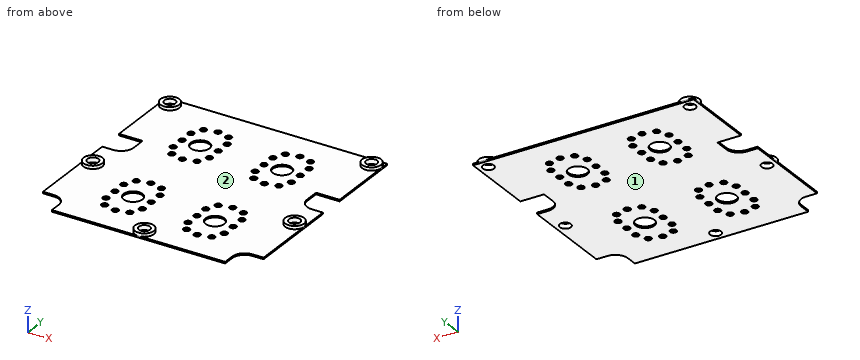
```python
from build123d import *

# Parameters (mm, degrees)
SKETCH1_W               = 70
SKETCH1_H               = 70
BOSS_EXTRUDE1_DEPTH     = 0.5
SKETCH2_R               = 3
CUT_EXTRUDE1_DEPTH      = 50.5
SKETCH3_R               = 1
CUT_EXTRUDE2_DEPTH      = 50.5
MIRROR2_COPY_1_SKETCH_R = 3
MIRROR2_COPY_1_DEPTH    = 50.5
MIRROR2_COPY_2_SKETCH_R = 1
MIRROR2_COPY_2_DEPTH    = 50.5
SKETCH4_R               = 3
BOSS_EXTRUDE2_DEPTH     = 1
SKETCH5_R               = 1.75
CUT_EXTRUDE3_DEPTH      = 50.520197899
SKETCH6_W               = 8.5
SKETCH6_H               = 8.5
CUT_EXTRUDE4_DEPTH      = 50.507575178
FILLET1_R               = 4
SKETCH7_R               = 3
BOSS_EXTRUDE3_DEPTH     = 1
SKETCH8_R               = 1.75
CUT_EXTRUDE5_DEPTH      = 50.520197899
FILLET1_OF_MIRROR3_R    = 4


with BuildPart() as part:
    # Sketch1 → Boss-Extrude1 (new body)
    with BuildSketch(Plane.XY):
        Rectangle(SKETCH1_W, SKETCH1_H)
    extrude(amount=BOSS_EXTRUDE1_DEPTH)

    # Sketch2 → Cut-Extrude1 (cut, through all)
    with BuildSketch(Plane.XY.offset(0.5)):
        with Locations((-13, 17)):
            Circle(SKETCH2_R)
    cut_extrude1 = extrude(amount=-CUT_EXTRUDE1_DEPTH, mode=Mode.SUBTRACT)

    # Sketch3 → Cut-Extrude2 (cut, through all)
    with BuildSketch(Plane.XY.offset(0.5)):
        with Locations((-7.25, 21.5)):
            Circle(SKETCH3_R)
        with Locations((-7.25, 17)):
            Circle(SKETCH3_R)
        with Locations((-7.25, 12.5)):
            Circle(SKETCH3_R)
        with Locations((-9, 9)):
            Circle(SKETCH3_R)
        with Locations((-9, 25)):
            Circle(SKETCH3_R)
        with Locations((-13, 26)):
            Circle(SKETCH3_R)
        with Locations((-13, 8)):
            Circle(SKETCH3_R)
        with Locations(Location((-17, 9, 0), (0, 0, 180))):
            Circle(SKETCH3_R)
        with Locations(Location((-18.75, 12.5, 0), (0, 0, 180))):
            Circle(SKETCH3_R)
        with Locations(Location((-18.75, 17, 0), (0, 0, 180))):
            Circle(SKETCH3_R)
        with Locations(Location((-18.75, 21.5, 0), (0, 0, 180))):
            Circle(SKETCH3_R)
        with Locations(Location((-17, 25, 0), (0, 0, 180))):
            Circle(SKETCH3_R)
    cut_extrude2 = extrude(amount=-CUT_EXTRUDE2_DEPTH, mode=Mode.SUBTRACT)

    # Mirror1: Cut-Extrude1, Cut-Extrude2 across plane
    add(cut_extrude1.mirror(Plane(origin=(0, 0, 0), x_dir=(0, 0, 1), z_dir=(1, 0, 0))), mode=Mode.SUBTRACT)
    add(cut_extrude2.mirror(Plane(origin=(0, 0, 0), x_dir=(0, 0, 1), z_dir=(1, 0, 0))), mode=Mode.SUBTRACT)

    # Mirror2: Cut-Extrude1, Cut-Extrude2 across plane
    add(cut_extrude1.mirror(Plane.ZX), mode=Mode.SUBTRACT)
    add(cut_extrude2.mirror(Plane.ZX), mode=Mode.SUBTRACT)

    # Mirror2 copy 1 sketch → Mirror2 copy 1 (cut, through all)
    with BuildSketch(Plane(origin=(0, 0, 0.5), x_dir=(-1, 0, 0), z_dir=(0, 0, 1))):
        with Locations((-13, 17)):
            Circle(MIRROR2_COPY_1_SKETCH_R)
    extrude(amount=-MIRROR2_COPY_1_DEPTH, mode=Mode.SUBTRACT)

    # Mirror2 copy 2 sketch → Mirror2 copy 2 (cut, through all)
    with BuildSketch(Plane(origin=(0, 0, 0.5), x_dir=(-1, 0, 0), z_dir=(0, 0, 1))):
        with Locations((-7.25, 21.5)):
            Circle(MIRROR2_COPY_2_SKETCH_R)
        with Locations((-7.25, 17)):
            Circle(MIRROR2_COPY_2_SKETCH_R)
        with Locations((-7.25, 12.5)):
            Circle(MIRROR2_COPY_2_SKETCH_R)
        with Locations((-9, 9)):
            Circle(MIRROR2_COPY_2_SKETCH_R)
        with Locations((-9, 25)):
            Circle(MIRROR2_COPY_2_SKETCH_R)
        with Locations((-13, 26)):
            Circle(MIRROR2_COPY_2_SKETCH_R)
        with Locations((-13, 8)):
            Circle(MIRROR2_COPY_2_SKETCH_R)
        with Locations(Location((-17, 9, 0), (0, 0, 180))):
            Circle(MIRROR2_COPY_2_SKETCH_R)
        with Locations(Location((-18.75, 12.5, 0), (0, 0, 180))):
            Circle(MIRROR2_COPY_2_SKETCH_R)
        with Locations(Location((-18.75, 17, 0), (0, 0, 180))):
            Circle(MIRROR2_COPY_2_SKETCH_R)
        with Locations(Location((-18.75, 21.5, 0), (0, 0, 180))):
            Circle(MIRROR2_COPY_2_SKETCH_R)
        with Locations(Location((-17, 25, 0), (0, 0, 180))):
            Circle(MIRROR2_COPY_2_SKETCH_R)
    extrude(amount=-MIRROR2_COPY_2_DEPTH, mode=Mode.SUBTRACT)

    # Sketch4 → Boss-Extrude2 (add)
    with BuildSketch(Plane.XY.offset(0.5)):
        with Locations(Location((-32, 32, 0), (0, 0, 180))):
            Circle(SKETCH4_R)
        with Locations(Location((-32, -7, 0), (0, 0, 180))):
            Circle(SKETCH4_R)
    boss_extrude2 = extrude(amount=BOSS_EXTRUDE2_DEPTH)

    # Sketch5 → Cut-Extrude3 (cut, through all)
    with BuildSketch(Plane.XY.offset(1.5)):
        with Locations((-32, 32)):
            Circle(SKETCH5_R)
        with Locations((-32, -7)):
            Circle(SKETCH5_R)
    cut_extrude3 = extrude(amount=-CUT_EXTRUDE3_DEPTH, mode=Mode.SUBTRACT)

    # Sketch6 → Cut-Extrude4 (cut, through all)
    with BuildSketch(Plane.XY.offset(0.5)):
        with Locations((-31.75, -31.75)):
            Rectangle(SKETCH6_W, SKETCH6_H)
        with Locations((-31.75, 6.75)):
            Rectangle(SKETCH6_W, SKETCH6_H)
    cut_extrude4 = extrude(amount=-CUT_EXTRUDE4_DEPTH, mode=Mode.SUBTRACT)

    # Fillet1
    fillet1_edges = [part.edges().sort_by_distance(p)[0] for p in [
        (-27.5, -27.5, 0.25),
        (-27.5, 2.5, 0.25),
    ]]
    fillet(fillet1_edges, radius=FILLET1_R)

    # Sketch7 → Boss-Extrude3 (add)
    with BuildSketch(Plane.XY.offset(0.5)):
        with Locations(Location((0, -32, 0), (0, 0, 270))):
            Circle(SKETCH7_R)
    extrude(amount=BOSS_EXTRUDE3_DEPTH)

    # Sketch8 → Cut-Extrude5 (cut, through all)
    with BuildSketch(Plane.XY.offset(1.5)):
        with Locations((0, -32)):
            Circle(SKETCH8_R)
    extrude(amount=-CUT_EXTRUDE5_DEPTH, mode=Mode.SUBTRACT)

    # Mirror3: Boss-Extrude2, Cut-Extrude3, Cut-Extrude4 across plane
    add(boss_extrude2.mirror(Plane(origin=(0, 0, 0), x_dir=(0, 0, 1), z_dir=(1, 0, 0))))
    add(cut_extrude3.mirror(Plane(origin=(0, 0, 0), x_dir=(0, 0, 1), z_dir=(1, 0, 0))), mode=Mode.SUBTRACT)
    add(cut_extrude4.mirror(Plane(origin=(0, 0, 0), x_dir=(0, 0, 1), z_dir=(1, 0, 0))), mode=Mode.SUBTRACT)

    # Fillet1 of Mirror3
    fillet1_of_mirror3_edges = [part.edges().sort_by_distance(p)[0] for p in [
        (27.5, -27.5, 0.25),
        (27.5, 2.5, 0.25),
    ]]
    fillet(fillet1_of_mirror3_edges, radius=FILLET1_OF_MIRROR3_R)


solid = part.part
```
Here's how the part is built. I have some questions about the finished solid (model axes, mm). Face numbers are marked on the shaded views. Give positions to 0.01 mm unless a question says otherwise; leave off trailing zeros. Write each loop counter-clockwise with the first axis right and the second up, starting at its lowest first coordinate (ties: lowest second). Pieces come first, ordered by that corner, then holes. Notation, with made-up numbers: (35, -2.5) -> (79, -2.5) arc R5 ccw to (79, 3.5) -> close; hole circle Ø5 at (-34.5, -18.5). An arc over 180 degrees is marked (long way). Use one line per item in the form item = value.
1) I'm going to push a flat-ended pin straight in: pin 1 (2.5 mm diameter, centred on x = 18.75, y = 17, fed in from +Z). Where does the tip first touch, or does it pass through?
Verdict:
pin_1 = 0.5
2) Suppose I cut it at A-A (x = -13). Please give me the cut outline in (y, z), and give its area (3 significant figures).
Verdict:
outline = (-35, 0) -> (-27, 0) -> (-27, 0.5) -> (-35, 0.5) -> close; (-25, 0) -> (-20, 0) -> (-20, 0.5) -> (-25, 0.5) -> close; (-14, 0) -> (-9, 0) -> (-9, 0.5) -> (-14, 0.5) -> close; (-7, 0) -> (7, 0) -> (7, 0.5) -> (-7, 0.5) -> close; (9, 0) -> (14, 0) -> (14, 0.5) -> (9, 0.5) -> close; (20, 0) -> (25, 0) -> (25, 0.5) -> (20, 0.5) -> close; (27, 0) -> (35, 0) -> (35, 0.5) -> (27, 0.5) -> close
area = 25.0 mm2
3) Suppose I cut it at C-C (z = 0.25). Give the number of separate pieces and of enclosed holes in the cut face, and give its area (3 significant figures).
Verdict:
separate_pieces = 1
enclosed_holes = 57
area = 4,360 mm2
4) If I drill on L1, parallel to Y at x = -32, z = 0.3; L2, parallel to Z at x = -16.5, y = -14; L3, parallel to X at y = -8, z = 1, over which ranges is the centre line in solid material (lowest first)? Write a range as [from, to].
Verdict:
L1 = [-27.5, -8.75], [-5.25, 2.5], [11, 30.25], [33.75, 35]
L2 = [0, 0.5]
L3 = [-34.83, -33.44], [-30.56, -29.17], [29.17, 30.56], [33.44, 34.83]
5) We'd pull the mould along X, two halves only. Please class the marked faces 1 and 2: +X half, -X half, draft (parallel to the pull), parting line (faces both ways), or undercut.
Verdict:
face_1 = draft
face_2 = undercut
6) Suppose I cut it at B-B (y = 21.5). Please give me the cut outline in (x, z), and give its area (3 significant figures).
Verdict:
outline = (-35, 0) -> (-19.75, 0) -> (-19.75, 0.5) -> (-35, 0.5) -> close; (-17.75, 0) -> (-8.25, 0) -> (-8.25, 0.5) -> (-17.75, 0.5) -> close; (-6.25, 0) -> (6.25, 0) -> (6.25, 0.5) -> (-6.25, 0.5) -> close; (8.25, 0) -> (17.75, 0) -> (17.75, 0.5) -> (8.25, 0.5) -> close; (19.75, 0) -> (35, 0) -> (35, 0.5) -> (19.75, 0.5) -> close
area = 31.0 mm2
7) Suppose I cut it at D-D (x = -21). Please give me the cut outline in (y, z), and give its area (3 significant figures).
Verdict:
outline = (-35, 0) -> (35, 0) -> (35, 0.5) -> (-35, 0.5) -> close
area = 35.0 mm2
